from build123d import *

# Parameters (mm, degrees)
BOSS_EXTRUDE1_DEPTH            = 6.35
CHAMFER1_SIZE                  = 0.508
FILLET1_R                      = 1.5875
M4X0_7_TAPPED_HOLE2_D          = 3.3
M3X0_5_TAPPED_HOLE1_AT_2_COUNT = 2
M3X0_5_TAPPED_HOLE1_AT_2_PITCH = 60.9
CIRPATTERN1_COUNT              = 4
SKETCH9_R                      = 1.5875
CUT_EXTRUDE2_DEPTH             = 71.290984486
CUT_EXTRUDE3_DEPTH             = 71.290984486
CIRPATTERN2_COUNT              = 4


with BuildPart() as part:
    # Sketch1 → Boss-Extrude1 (new body)
    with BuildSketch(Plane(origin=(0, 0, 0), x_dir=(1, 0, 0), z_dir=(0, 1, 0))):
        Polygon((-47.9125, 22.5125), (-49.5, 22.5125), (-49.5, -22.5125), (-47.9125, -22.5125), (-47.9125, -47.9125), (-22.5125, -47.9125), (-22.5125, -49.5), (22.5125, -49.5), (22.5125, -47.9125), (47.9125, -47.9125), (47.9125, -22.5125), (49.5, -22.5125), (49.5, 22.5125), (47.9125, 22.5125), (47.9125, 47.9125), (22.5125, 47.9125), (22.5125, 49.5), (-22.5125, 49.5), (-22.5125, 47.9125), (-47.9125, 47.9125), align=None)
    extrude(amount=BOSS_EXTRUDE1_DEPTH)

    # Chamfer1
    chamfer1_edges = [part.edges().sort_by_distance(p)[0] for p in [
        (-47.9125, 3.175, -47.9125),
        (47.9125, 3.175, -47.9125),
        (47.9125, 3.175, 47.9125),
        (-47.9125, 3.175, 47.9125),
    ]]
    chamfer(chamfer1_edges, length=CHAMFER1_SIZE)

    # Fillet1
    fillet1_edges = [part.edges().sort_by_distance(p)[0] for p in [
        (-47.9125, 3.175, -22.5125),
        (-22.5125, 3.175, -47.9125),
        (22.5125, 3.175, -47.9125),
        (47.9125, 3.175, -22.5125),
        (47.9125, 3.175, 22.5125),
        (22.5125, 3.175, 47.9125),
        (-22.5125, 3.175, 47.9125),
        (-47.9125, 3.175, 22.5125),
    ]]
    fillet(fillet1_edges, radius=FILLET1_R - 0.0001)  # a hair under: the kernel refuses the full size

    # M4x0.7 Tapped Hole2 (through all)
    with Locations(Plane(origin=(0, 0, 0), x_dir=(-1, 0, 0), z_dir=(0, -1, 0))):
        with Locations((-45.25, 45.25), (45.25, 45.25), (45.25, -45.25), (-45.25, -45.25)):
            Hole(M4X0_7_TAPPED_HOLE2_D / 2)

    # Sketch7 → M3x0.5 Tapped Hole1 (revolve, cut)
    with BuildSketch(Plane(origin=(-30.45, 3.175, 47.9125), x_dir=(0, -1, 0), z_dir=(1, 0, 0))):
        Polygon((0, 0), (0, 8.371075774), (1.25, 7.62), (1.25, 0), align=None)
    m3x0_5_tapped_hole1 = revolve(axis=Axis((-30.45, 3.175, 54.2625), (0, 0, -1)), mode=Mode.SUBTRACT)

    # M3x0.5 Tapped Hole1 at 2: M3x0.5 Tapped Hole1 ×2
    with Locations(*[(i * M3X0_5_TAPPED_HOLE1_AT_2_PITCH, 0, 0) for i in range(1, M3X0_5_TAPPED_HOLE1_AT_2_COUNT)]):
        add(m3x0_5_tapped_hole1, mode=Mode.SUBTRACT)

    # CirPattern1: M3x0.5 Tapped Hole1 ×4 about axis
    cirpattern1_axis = Axis((0, -0.3175, 0), (0, 1, 0))
    for i in range(1, CIRPATTERN1_COUNT):
        add(m3x0_5_tapped_hole1.rotate(cirpattern1_axis, i * 360 / CIRPATTERN1_COUNT), mode=Mode.SUBTRACT)

    # CirPattern1 copy 1 sketch → CirPattern1 copy 1 (revolve, cut)
    with BuildSketch(Plane(origin=(47.9125, 3.175, -30.45), x_dir=(0, -1, 0), z_dir=(0, 0, -1))):
        Polygon((0, 0), (0, 8.371075774), (1.25, 7.62), (1.25, 0), align=None)
    revolve(axis=Axis((54.2625, 3.175, -30.45), (-1, 0, 0)), mode=Mode.SUBTRACT)

    # CirPattern1 copy 2 sketch → CirPattern1 copy 2 (revolve, cut)
    with BuildSketch(Plane(origin=(-30.45, 3.175, -47.9125), x_dir=(0, -1, 0), z_dir=(-1, 0, 0))):
        Polygon((0, 0), (0, 8.371075774), (1.25, 7.62), (1.25, 0), align=None)
    revolve(axis=Axis((-30.45, 3.175, -54.2625), (0, 0, 1)), mode=Mode.SUBTRACT)

    # CirPattern1 copy 3 sketch → CirPattern1 copy 3 (revolve, cut)
    with BuildSketch(Plane(origin=(-47.9125, 3.175, 30.45), x_dir=(0, -1, 0), z_dir=(0, 0, 1))):
        Polygon((0, 0), (0, 8.371075774), (1.25, 7.62), (1.25, 0), align=None)
    revolve(axis=Axis((-54.2625, 3.175, 30.45), (1, 0, 0)), mode=Mode.SUBTRACT)

    # Sketch9 → Cut-Extrude2 (cut, through all)
    with BuildSketch(Plane(origin=(0, 6.35, 0), x_dir=(1, 0, 0), z_dir=(0, 1, 0))):
        with Locations(Location((-40.005, -42.926, 0), (0, 0, 270))):
            Circle(SKETCH9_R)
        with Locations(Location((40.005, -42.926, 0), (0, 0, 270))):
            Circle(SKETCH9_R)
        with Locations(Location((37.465, 42.8625, 0), (0, 0, 270))):
            Circle(SKETCH9_R)
        with Locations(Location((-36.195, 42.8625, 0), (0, 0, 270))):
            Circle(SKETCH9_R)
    extrude(amount=-CUT_EXTRUDE2_DEPTH, mode=Mode.SUBTRACT)

    # Sketch15 → M3x0.5 Tapped Hole3 (revolve, cut)
    with BuildSketch(Plane(origin=(0, 6.35, 46.325), x_dir=(0, 0, 1), z_dir=(1, 0, 0))):
        Polygon((0, 0), (0, 8.371075774), (1.25, 7.62), (1.25, 0), align=None)
    m3x0_5_tapped_hole3 = revolve(axis=Axis((0, 12.7, 46.325), (0, -1, 0)), mode=Mode.SUBTRACT)

    # Sketch16 → Cut-Extrude3 (cut, through all)
    with BuildSketch(Plane(origin=(0, 6.35, 0), x_dir=(1, 0, 0), z_dir=(0, 1, 0))):
        with BuildLine():
            ThreePointArc((-43.15, -24.1), (-37.570384182, -37.570384182), (-24.1, -43.15))
            Line((-24.1, -43.15), (24.1, -43.15))
            ThreePointArc((24.1, -43.15), (37.570384182, -37.570384182), (43.15, -24.1))
            Line((43.15, -24.1), (43.15, 24.1))
            ThreePointArc((43.15, 24.1), (37.570384182, 37.570384182), (24.1, 43.15))
            Line((24.1, 43.15), (-24.1, 43.15))
            ThreePointArc((-24.1, 43.15), (-37.570384182, 37.570384182), (-43.15, 24.1))
            Line((-43.15, 24.1), (-43.15, -24.1))
        make_face()
    extrude(amount=-CUT_EXTRUDE3_DEPTH, mode=Mode.SUBTRACT)

    # CirPattern2: M3x0.5 Tapped Hole3 ×4 about axis
    cirpattern2_axis = Axis((0, 0, 0), (0, 1, 0))
    for i in range(1, CIRPATTERN2_COUNT):
        add(m3x0_5_tapped_hole3.rotate(cirpattern2_axis, i * 360 / CIRPATTERN2_COUNT), mode=Mode.SUBTRACT)


solid = part.part
Read the model definition and answer for the solid it produces. Units are mm, in the model's axes. A direction names the side the tool comes from. Coordinates: 2 decimals unless noted, no trailing zeros. Loops run counter-clockwise (first coordinate to the right, second up) from the corner with the lowest first, then second, coordinate; pieces in that order, holes last.
Q1. Each of these flat-tipped pins is pushed along its axis until it touches: pin 1 Ø1.9 at (x, y) = (-34, 4) entering from +Z; pin 2 Ø1.5 at (y, z) = (1, 30.5) entering from +X; pin 3 Ø3 at (x, y) = (-30.45, 3.175) entering from -Z. Where does it stop, or does it pass through?
Q2. The part is cut by section B-B on x = 0. Write down the section's boundary in (y, z) (3 decimals).
Q3. The part is cut by section C-C on z = 0. Write down the section's boundary in (x, y) (3 decimals).
Q4. Which of the six approach directions +Z, -Z, +X, -X, +Y, -Y give full straight-line access (tool end or side, diameter ignored) to faces 4 (the face through (-37.42, 3.22, -37.72)), 5 (the face through (31.5, 2.5, -44.8)), 6 (the face through (-36, 3, 47.912)), 7 (the face through (44.78, 3.45, -31.67)), 8 (the face through (47.912, 3, -36))?
Q5. The mould has two halves that part along Z. Classify faces 1 (the face through (0, 3, -49.5)), 2 (the face through (0, 3, 49.5)), 3 (the face through (-44.8, 2.5, -31.5)): +Z half, -Z half, draft (parallel to the pull), parting line (faces both ways), or undercut.
Q6. The part is cut by section A-A on z = -17. Write down the section's boundary in (x, y).
Q7. Consider probe 1 along X at (y, z) = (2.5, 10); probe 2 along X at (y, z) = (2.25, -0.5). Determine where each line is inside the solid, lowest interval first.
Q8. The part is cut by section D-D on x = 11. Write down the section's boundary in (y, z), and give its area (3 significant figures).
Results below:
1. pin 1: stops at z = 47.91
1. pin 2: stops at x = 47.91
1. pin 3: stops at z = -47.91
2. outline: (0, -49.5) - (6.35, -49.5) - (6.35, -47.575) - (0, -47.575) - close; (0, -45.075) - (6.35, -45.075) - (6.35, -43.15) - (0, -43.15) - close; (0, 43.15) - (6.35, 43.15) - (6.35, 45.075) - (0, 45.075) - close; (0, 47.575) - (6.35, 47.575) - (6.35, 49.5) - (0, 49.5) - close
3. outline: (-49.5, 0) - (-47.575, 0) - (-47.575, 6.35) - (-49.5, 6.35) - close; (-45.075, 0) - (-43.15, 0) - (-43.15, 6.35) - (-45.075, 6.35) - close; (43.15, 0) - (45.075, 0) - (45.075, 6.35) - (43.15, 6.35) - close; (47.575, 0) - (49.5, 0) - (49.5, 6.35) - (47.575, 6.35) - close
4. face 4: +Y, -Y
4. face 5: +Z, -Z
4. face 6: +Z, -X, +Y, -Y
4. face 7: +X, -X
4. face 8: -Z, +X, +Y, -Y
5. face 1: -Z half
5. face 2: +Z half
5. face 3: undercut
6. outline: (-49.5, 0) - (-43.15, 0) - (-43.15, 6.35) - (-49.5, 6.35) - close; (43.15, 0) - (49.5, 0) - (49.5, 6.35) - (43.15, 6.35) - close
7. probe 1: x = -49.5 to -43.15, 43.15 to 49.5
7. probe 2: x = -49.5 to -47.47, -45.18 to -43.15, 43.15 to 45.18, 47.47 to 49.5
8. outline: (0, -49.5) - (6.35, -49.5) - (6.35, -43.15) - (0, -43.15) - close; (0, 43.15) - (6.35, 43.15) - (6.35, 49.5) - (0, 49.5) - close
8. area: 80.6 mm2
